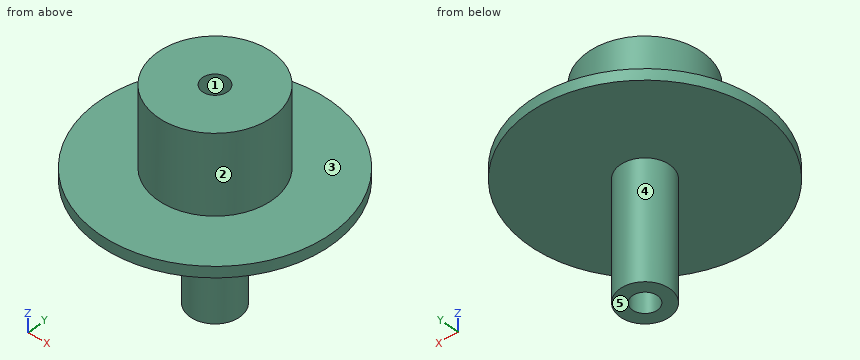
```python
from build123d import *

# Parameters (mm, degrees)
SKETCH2_R          = 28.5
CUT_EXTRUDE1_DEPTH = 604.380476979


with BuildPart() as part:
    # Sketch1 → Revolve1 (revolve)
    with BuildSketch(Plane(origin=(0, 0, 0), x_dir=(0, 0, -1), z_dir=(1, 0, 0)), mode=Mode.PRIVATE) as revolve1_sk:
        Polygon((0, 0), (0, 130), (180, 130), (180, 264), (205, 264), (205, 56.5), (474, 56.5), (474, 0), align=None)
    revolve(revolve1_sk.sketch.rotate(Axis((0, 0, 0), (0, 0, -1)), 180), axis=Axis((0, 0, 0), (0, 0, -1)))

    # Sketch2 → Cut-Extrude1 (cut, through all)
    with BuildSketch(Plane.XY):
        Circle(SKETCH2_R)
    extrude(amount=-CUT_EXTRUDE1_DEPTH, mode=Mode.SUBTRACT)


solid = part.part
```
Input: part model. Units: mm. Frame: model coordinates. Face numbers are marked on the shaded views. A direction names the side the tool comes from. Give positions to 0.01 mm unless a question says otherwise; leave off trailing zeros. Order: outer loops, then holes, each group sorted by start corner. A loop starts at its lowest first (then second) coordinate and runs counter-clockwise, first axis right, second up. Notation, with made-up numbers: (23, -9) - (51, -9) arc R22 cw to (51, 18) - close; hole circle Ø11 at (-37, -6). An arc over 180 degrees is marked (long way). Use a Markdown table: item, result.
(1) Line query: line 1 (Z direction, x = 231, y = -58); line 2 (X direction, y = -24, z = -21); line 3 (Z direction, x = 71.5, y = 25.5). Output: solid intervals per line, ascending. Write a range as from..to.
Computed values:
| item | result |
|---|---|
| line 1 | z = -205..-180 |
| line 2 | x = -127.77..-15.37, 15.37..127.77 |
| line 3 | z = -205..0 |
(2) Section query D-D (y = -90). Output: boundary loops of the cut face in (x, z).
Computed values:
| item | result |
|---|---|
| outline | (-248.19, -205) - (248.19, -205) - (248.19, -180) - (93.81, -180) - (93.81, 0) - (-93.81, 0) - (-93.81, -180) - (-248.19, -180) - close |
(3) Section query A-A (y = 0). Output: boundary loops of the cut face in (x, z), then the cut area to 3 significant figures.
Computed values:
| item | result |
|---|---|
| outline | (-264, -205) - (-56.5, -205) - (-56.5, -474) - (-28.5, -474) - (-28.5, 0) - (-130, 0) - (-130, -180) - (-264, -180) - close; (28.5, -474) - (56.5, -474) - (56.5, -205) - (264, -205) - (264, -180) - (130, -180) - (130, 0) - (28.5, 0) - close |
| area | 63,400 mm2 |
(4) Pin query (flat end, axial travel): pin 1 (12 mm diameter, centred on x = -66.5, z = -381.5, fed in from +Y); pin 2 (4 mm diameter, centred on x = 33.5, y = -51.5, fed in from -Z); pin 3 (4 mm diameter, centred on y = -22.5, z = -159, fed in from +X); pin 4 (3 mm diameter, centred on x = -118, y = -107, fed in from +Z). Return the tip coordinate at first contact, or that it passes through.
Computed values:
| item | result |
|---|---|
| pin 1 | passes through |
| pin 2 | stops at z = -205 |
| pin 3 | stops at x = 128.37 |
| pin 4 | stops at z = -180 |
(5) Section query C-C (z = -126.5). Output: boundary loops of the cut face in (x, y), then the cut area to 3 significant figures.
Computed values:
| item | result |
|---|---|
| outline | circle Ø260 at (0, 0); hole circle Ø57 at (0, 0) |
| area | 50,500 mm2 |
(6) Draft query along X for the marked faces 1, 2 and 3. Return one class per face: released by +X, released by -X, zero draft, split by the parting line, or undercut.
Computed values:
| item | result |
|---|---|
| face 1 | undercut |
| face 2 | split by the parting line |
| face 3 | zero draft |
(7) Access query for the marked faces 4 and 5. Directions: +Z, -Z, +X, -X, +Y, -Y. A direction counts if a zero-diameter tool reaches every point of the face in a straight line with its end or side. Return the directions, or none.
Computed values:
| item | result |
|---|---|
| face 4 | -Z |
| face 5 | -Z, +X, -X, +Y, -Y |
